from build123d import *

# Parameters (mm, degrees)
BOSS_EXTRUDE1_DEPTH = 1.5
FILLET1_R           = 2
CUT_EXTRUDE1_DEPTH  = 10


with BuildPart() as part:
    # Sketch1 → Boss-Extrude1 (new body)
    with BuildSketch(Plane.XY):
        Polygon((0, 0), (177, 0), (177, 186), (105, 186), (105, 166), (72, 166), (72, 186), (0, 186), align=None)
    extrude(amount=BOSS_EXTRUDE1_DEPTH)

    # Fillet1
    fillet1_edges = [part.edges().sort_by_distance(p)[0] for p in [
        (0, 186, 0.75),
        (72, 186, 0.75),
        (72, 166, 0.75),
        (105, 166, 0.75),
        (105, 186, 0.75),
        (177, 186, 0.75),
        (177, 0, 0.75),
        (0, 0, 0.75),
    ]]
    fillet(fillet1_edges, radius=FILLET1_R)

    # Sketch2 → Cut-Extrude1 (cut)
    with BuildSketch(Plane(origin=(0, 0, 0), x_dir=(-1, 0, 0), z_dir=(0, 0, -1))):
        with BuildLine():
            Line((-126, 99.5), (-51, 99.5))
            ThreePointArc((-51, 99.5), (-31, 79.5), (-51, 59.5))
            Line((-51, 59.5), (-126, 59.5))
            ThreePointArc((-126, 59.5), (-146, 79.5), (-126, 99.5))
        make_face()
    extrude(amount=-CUT_EXTRUDE1_DEPTH, mode=Mode.SUBTRACT)


solid = part.part
Geometry: final body of the model. Coordinates: model frame, mm. A direction names the side the tool comes from. Coordinates: 2 decimals unless noted, no trailing zeros. Order: outer loops, then holes, each group sorted by start corner. A loop starts at its lowest first (then second) coordinate and runs counter-clockwise, first axis right, second up. Notation, with made-up numbers: M 81.25,-12.5 L 95.25,-12.5 A23 cw 95.25,9.5 Z; hole C -23,11.25 d5. An arc over 180 degrees is marked long. One line per question, with ' | ' between items. Start each with the question number.
Item 1: Ray query, probe 1 along X at (y, z) = (79.5, 1.25); probe 2 along Y at (x, z) = (67, 1.05); probe 3 along Y at (x, z) = (98, 0.3). Return the intervals inside material, ascending. Write a range as [from, to].
Item 2: Cut plane C-C, the plane y = 79.5. Return the cut outline in (x, z), then the cut area to 3 significant figures.
Item 3: Cut plane B-B, the plane z = 1.25. Return the cut outline in (x, y), then the cut area to 3 significant figures.
Item 4: Set-up query: faces 3 (the flat face through (87, 115, 1.5)), 4 (the cylindrical face through (31.005, 79.94, 0.74)). Return all of +Z, -Z, +X, -X, +Y, -Y with unobstructed straight access to the full face (end or side cutting, diameter ignored); none if empty.
Item 5: Cut plane A-A, the plane x = 81. Return the cut outline in (y, z), then the cut area to 3 significant figures.
Item 6: Draft query along X for faces 1 (the flat face through (87, 115, 0)), 2 (the cylindrical face through (145.995, 79.06, 0.74)). Return one class per face: released by +X, released by -X, zero draft, split by the parting line, or undercut.
A:
1) probe 1: x = [0, 31], [146, 177] | probe 2: y = [0, 59.5], [99.5, 186] | probe 3: y = [0, 59.5], [99.5, 166]
2) outline: M 0,0 L 31,0 L 31,1.5 L 0,1.5 Z; M 146,0 L 177,0 L 177,1.5 L 146,1.5 Z | area: 93.0 mm2
3) outline: M 0,2 A2 ccw 2,0 L 175,0 A2 ccw 177,2 L 177,184 A2 ccw 175,186 L 107,186 A2 ccw 105,184 L 105,168 A2 cw 103,166 L 74,166 A2 cw 72,168 L 72,184 A2 ccw 70,186 L 2,186 A2 ccw 0,184 Z; hole M 51,59.5 L 126,59.5 A20 ccw 126,99.5 L 51,99.5 A20 ccw Z | area: 28,000 mm2
4) face 3: +Z, +X, -X, +Y, -Y | face 4: +Z, -Z
5) outline: M 0,0 L 59.5,0 L 59.5,1.5 L 0,1.5 Z; M 99.5,0 L 166,0 L 166,1.5 L 99.5,1.5 Z | area: 189 mm2
6) face 1: zero draft | face 2: undercut
